```python
from build123d import *

# Parameters (mm, degrees)
F0_R        = 35
F1_DEPTH    = 180
F2_R        = 15
F3_DEPTH    = 10
F4_SIZE     = 4.99999
F5_R        = 17.6680128579
F6_DEPTH    = 25
F7_R        = 5
F8_R        = 5
F9_S5_R     = 17.6680128579
F9_T6_DEPTH = 53
F10_T       = 2.5


# Not quite as in the source:
# - a fillet or chamfer that OpenCascade refuses, or shapes differently, is made with other operations: its cross-section is extruded or revolved along the edge and cut away or added
# - a fillet or chamfer is up to 0.001 mm smaller than in the source, because OpenCascade refuses the exact size
# - a shell that OpenCascade refuses in one call is made with other operations: the cavity is built on its own and cut out


with BuildPart() as f1:
    # F0 (on Top) → F1 (new body)
    with BuildSketch(Plane.XY):
        Circle(F0_R)
    extrude(amount=F1_DEPTH)

    # F2 (on face) → F3 (cut)
    with BuildSketch(Plane(origin=(0, 0, 0), x_dir=(1, 0, 0), z_dir=(0, 0, -1))):
        Circle(F2_R)
    extrude(amount=-F3_DEPTH, mode=Mode.SUBTRACT)

    # F4 (size 5 in the source; OpenCascade refuses exactly that, so slightly less here)
    f4_edges = [f1.edges().sort_by_distance(p)[0] for p in [
        (-15, 0, 10),
        (-15, 0, 0),
    ]]
    chamfer(f4_edges, length=F4_SIZE)

    # F5 (on face) → F6 (join)
    with BuildSketch(Plane.XY.offset(180)):
        Circle(F5_R)
    extrude(amount=F6_DEPTH)

    # F7
    f7_edges = [f1.edges().sort_by_distance(p)[0] for p in [
        (-17.668013, 0, 205),
    ]]
    fillet(f7_edges, radius=F7_R)

    # F8
    f8_edges = [f1.edges().sort_by_distance(p)[0] for p in [
        (-35, 0, 0),
    ]]
    fillet(f8_edges, radius=F8_R)

    # F9: chamfer of 25 on 1 edges, made by hand


with BuildPart() as f9_tool2:
    # F9_s3 → F9_t4 (revolve)
    with BuildSketch(Plane.XZ):
        Polygon((35, 155), (10, 180), (35, 180), align=None)
    revolve(axis=Axis((0, 0, 180), (0, 0, 1)))

    # F9_s5 → F9_t6 (cut, symmetric)
    with BuildSketch(Plane.XY.offset(167.5)):
        Circle(F9_S5_R)
    extrude(amount=F9_T6_DEPTH, both=True, mode=Mode.SUBTRACT)


with BuildPart() as f1_1:
    add(f1.part)

    # F9_t1: cut F9_tool2
    add(f9_tool2.part, mode=Mode.SUBTRACT)

    # F10: shell of thickness 2.5, made by hand


with BuildPart() as f10_core1:
    # F10_t2: copy of F1
    add(f1_1.part)

    # the walls: a layer under each face that stays
    f10_faces = [f10_core1.faces().sort_by_distance(p)[0] for p in [
        (-35, 0, 80),
        (-26.334006429, 0, 163.665993571),
        (-17.6680128579, 0, 186.165993571),
        (-16.2035467638, 0, 203.5355339059),
        (-33.5355339059, 0, 1.4644660941),
        (-20, -20, 0),
        (-17.499995, 0, 2.499995),
        (-15, 0, 5),
        (-12.500005, 0, 7.500005),
        (0, 0, 10),
    ]]
    thicken(f10_faces, amount=-F10_T, mode=Mode.SUBTRACT)

    # F10_s3 → F10_t4 (revolve, cut)
    with BuildSketch(Plane.XZ):
        Polygon((17.7106905274, 172.3496648116), (15.9002459049, 170.5642201891), (15.1680128579, 171.2964532362), (15.1680128579, 172.3319871421), align=None)
    revolve(axis=Axis((0, 0, 172.3319871421), (0, 0, 1)), mode=Mode.SUBTRACT)

    # F10_s5 → F10_t6 (revolve, cut)
    with BuildSketch(Plane.XZ):
        Polygon((14.9573223305, 4.9823323305), (17.5, 5.00001), (17.5, 6.0355439059), (16.767766953, 6.767776953), align=None)
    revolve(axis=Axis((0, 0, 5.00001), (0, 0, -1)), mode=Mode.SUBTRACT)

    # F10_s7 → F10_t8 (revolve, cut)
    with BuildSketch(Plane.XZ):
        Polygon((9.9823323305, 9.9573223305), (11.767776953, 11.767766953), (11.0355439059, 12.5), (10.00001, 12.5), align=None)
    revolve(axis=Axis((0, 0, 10), (0, 0, -1)), mode=Mode.SUBTRACT)


with BuildPart() as f1_2:
    add(f1_1.part)

    # what is left inside the walls is the cavity
    f10_cavity = [f10_core1.part.solids().sort_by_distance(p)[0] for p in [
        (-32.475, 0, 104.309644),
    ]]
    add(f10_cavity, mode=Mode.SUBTRACT)


solid = f1_2.part
```
Could you check a few things on this model? Use its own coordinates, in mm. A direction names the side the tool comes from. Round coordinates to 2 decimals unless told otherwise and drop trailing zeros. Order: outer loops, then holes, each group sorted by start corner. A loop starts at its lowest first (then second) coordinate and runs counter-clockwise, first axis right, second up. Notation, with made-up numbers: (48.5, 75.5) -> (100.5, 75.5) arc R9 cw to (100.5, 90.5) -> close; hole circle Ø9 at (45, 25). An arc over 180 degrees is marked (long way). One line per question, with ' | ' between items.
Q1. Which directions (+Z, -Z, +X, -X, +Y, -Y) give clear straight access to the entire face, cutting with the end or side of a thin tool? Please do faces 1 (the face through (-20.4, -6.2, 2.5)), 2 (the face through (0, 0, 10)), 3 (the face through (-3.83, -17.248, 186.36)).
Computed values:
face 1: none | face 2: -Z | face 3: +Z
Q2. If we section it at A-A on z = 42.5: Write out the boundary of the cut face in (x, y).
Computed values:
outline: circle Ø70 at (0, 0); hole circle Ø65 at (0, 0)
Q3. I'm going to push flat-ended pins straight in: pin 1 (10 mm diameter, centred on x = -18.5, z = 113.5, fed in from -Y); pin 2 (1 mm diameter, centred on x = 18.5, y = -18, fed in from +Z); pin 3 (18 mm diameter, centred on x = 0, y = 0, fed in from -Z). Where does each tip first touch, or does it pass through?
Computed values:
pin 1: y = -32.29 | pin 2: z = 164.69 | pin 3: z = 10
Q4. If I drill on line 1 (Y direction, x = 1, z = 74.5); line 2 (Y direction, x = 0, z = 5); line 3 (Z direction, x = -1, y = 3), over which ranges is the centre line in solid material (lowest first)? Write a range as from..to.
Computed values:
line 1: -34.99..-32.48, 32.48..34.99 | line 2: -35..-32.5, -18.54..-15, 15..18.54, 32.5..35 | line 3: 10..12.5
Q5. If we section it at B-B on z = 178: Write out the boundary of the cut face in (x, y), plus the area to 3 significant figures.
Computed values:
outline: circle Ø35.34 at (0, 0); hole circle Ø30.34 at (0, 0) | area: 258 mm²
Q6. We'd pull the mould along Y, two halves only. Please class faces 4 (the face through (20, -6, 0)), 5 (the face through (-28, -21, 79)), 6 (the face through (0, 0, 12.5)): released by +Y, released by -Y, zero draft, split by the parting line, or undercut.
Computed values:
face 4: zero draft | face 5: split by the parting line | face 6: undercut
